from build123d import *

# Parameters (mm, degrees)
F0_W     = 50
F0_H     = 950
F1_DEPTH = 100
F2_R     = 5
F3_T     = -4


with BuildPart() as f1:
    # F0 (on Top) → F1 (new body)
    with BuildSketch(Plane.XY):
        with Locations((-25, 475)):
            Rectangle(F0_W, F0_H)
    extrude(amount=F1_DEPTH)

    # F2
    f2_edges = [f1.edges().sort_by_distance(p)[0] for p in [
        (0, 475, 100),
        (-50, 475, 100),
        (0, 475, 0),
        (-50, 475, 0),
    ]]
    fillet(f2_edges, radius=F2_R)

    # F3
    f3_openings = [f1.faces().sort_by_distance(p)[0] for p in [
        (-25, 0, 50),
        (-25, 950, 50),
    ]]
    offset(amount=F3_T, openings=f3_openings)


solid = f1.part
Can you work these out from the model? Positions are in its coordinate system, mm. A direction names the side the tool comes from. Round coordinates to 2 decimals unless told otherwise and drop trailing zeros. Write each loop counter-clockwise with the first axis right and the second up, starting at its lowest first coordinate (ties: lowest second). Pieces come first, ordered by that corner, then holes. Notation, with made-up numbers: M -28.5,-27.5 L 13.5,-27.5 A6 cw 13.5,-23.5 Z; hole C 51.25,-5 d2. An arc over 180 degrees is marked long. Use a Markdown table: item, result.
Item 1: I want a section at A-A (z = 54). List the corners of the cut face in (x, y) for me.
Found:
| item | result |
|---|---|
| outline | M -50,0 L -46,0 L -46,950 L -50,950 Z; M -4,0 L 0,0 L 0,950 L -4,950 Z |
Item 2: I want a section at C-C (y = 582). List the corners of the cut face in (x, z) for me, and give its area (3 significant figures).
Found:
| item | result |
|---|---|
| outline | M -50,5 A5 ccw -45,0 L -5,0 A5 ccw 0,5 L 0,95 A5 ccw -5,100 L -45,100 A5 ccw -50,95 Z; hole M -46,5 A1 ccw -45,4 L -5,4 A1 ccw -4,5 L -4,95 A1 ccw -5,96 L -45,96 A1 ccw -46,95 Z |
| area | 1,120 mm2 |
Item 3: If I drill on line 1 along Z through (x, y) = (-23.5, 749.5); line 2 along X through (y, z) = (544.5, 21); line 3 along Z through (x, y) = (-2.5, 563.5), over which ranges is the centre line in solid material (lowest first)? Write a range as [from, to].
Found:
| item | result |
|---|---|
| line 1 | z = [0, 4], [96, 100] |
| line 2 | x = [-50, -46], [-4, 0] |
| line 3 | z = [0.67, 99.33] |
Item 4: I want a section at B-B (x = -26.5). List the corners of the cut face in (y, z) for me, and give its area (3 significant figures).
Found:
| item | result |
|---|---|
| outline | M 0,0 L 950,0 L 950,4 L 0,4 Z; M 0,96 L 950,96 L 950,100 L 0,100 Z |
| area | 7,600 mm2 |
Item 5: Which directions (+Z, -Z, +X, -X, +Y, -Y) give clear straight access to the entire face, cutting with the end or side of a thin tool? Please do faces 1 (the face through (-46, 468, 49)), 2 (the face through (0, 468, 49)).
Found:
| item | result |
|---|---|
| face 1 | +Y, -Y |
| face 2 | +Z, -Z, +X, +Y, -Y |
Item 6: We'd pull the mould along Z, two halves only. Please class faces 3 (the face through (-4, 468, 49)), 4 (the face through (-50, 468, 49)), 5 (the face through (-25, 482, 0)): released by +Z, released by -Z, zero draft, split by the parting line, or undercut.
Found:
| item | result |
|---|---|
| face 3 | undercut |
| face 4 | zero draft |
| face 5 | released by -Z |
